```python
from build123d import *

# Parameters (mm, degrees)
F0_W     = 96.4296718666
F0_H     = 58.42
F1_DEPTH = 25.4
F4_DEPTH = 254
F6_DEPTH = 12.7
F2_R     = 8.8980244031
F7_DEPTH = 254


# Not quite as in the source:
# - a pattern or mirror of a feature is missing from the dataset's text; its kind, count and spacing are read off the source's solid


with BuildPart() as f1:
    # F0 (on Front) → F1 (new body, symmetric)
    with BuildSketch(Plane.XZ):
        Rectangle(F0_W, F0_H)
    extrude(amount=F1_DEPTH, both=True)

    # F3 (on face) → F4 (cut)
    with BuildSketch(Plane.XZ.offset(25.4)):
        with BuildLine():
            Line((12.7, 29.21), (-12.7, 29.21))
            ThreePointArc((-12.7, 29.21), (0, 16.51), (12.7, 29.21))
        make_face()
    extrude(amount=-F4_DEPTH, mode=Mode.SUBTRACT)

    # F5 (on face) → F6 (join)
    with BuildSketch(Plane(origin=(0, 25.4, 0), x_dir=(-1, 0, 0), z_dir=(0, 1, 0))):
        with BuildLine():
            Line((-12.7, 29.21), (-25.4, 29.21))
            ThreePointArc((-25.4, 29.21), (0, 3.81), (25.4, 29.21))
            Line((25.4, 29.21), (12.7, 29.21))
            ThreePointArc((12.7, 29.21), (0, 16.51), (-12.7, 29.21))
        make_face()
    f6 = extrude(amount=F6_DEPTH)

    # F6_copies: F6 across plane
    add(f6.mirror(Plane(origin=(0, 0, 0), x_dir=(0, 0, -1), z_dir=(0, -1, 0))))

    # F2 (on face) → F7 (cut)
    with BuildSketch(Plane.XY.offset(29.21)):
        with Locations((35.2072529495, 0)):
            Circle(F2_R)
        with Locations((-35.2072529495, 0)):
            Circle(F2_R)
    extrude(amount=-F7_DEPTH, mode=Mode.SUBTRACT)


solid = f1.part
```
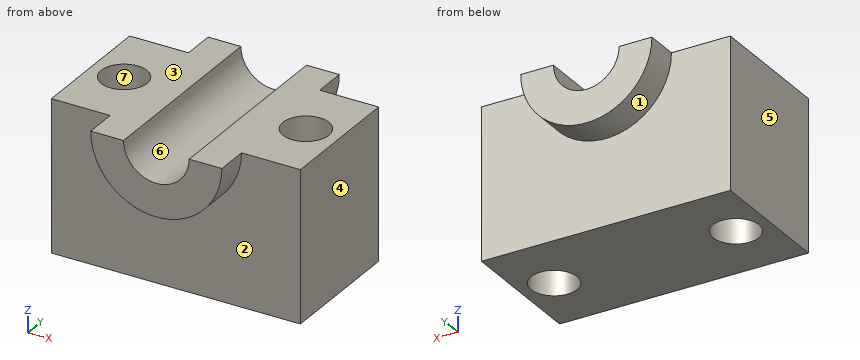
Check sheet for the modelled part. Datum: model origin and axes. Units: mm. Face numbers are marked on the shaded views. A direction names the side the tool comes from. Round coordinates to 2 decimals unless told otherwise and drop trailing zeros. Write each loop counter-clockwise with the first axis right and the second up, starting at its lowest first coordinate (ties: lowest second). Pieces come first, ordered by that corner, then holes. Notation, with made-up numbers: M 4,-10 L 35,-10 A29 cw 35,26 Z; hole C 46,38.5 d7. An arc over 180 degrees is marked long. Write item = value, one per line. Start each with the question number.
1. Section check D-D, the plane y = -20.5. Record the cut outline in (x, z).
2. Section check C-C, the plane x = 0. Record the cut outline in (y, z), then the cut area to 3 significant figures.
3. Gauge pin test, flat ends, axial feed: pin 1 (20.5 mm diameter, centred on x = -35.21, y = 0, fed in from -Z); pin 2 (8 mm diameter, centred on x = -35.5, y = -2, fed in from -Z); pin 3 (2 mm diameter, centred on y = -27, z = 6.5, fed in from +X); pin 4 (4 mm diameter, centred on x = 8, y = 23.5, fed in from +Z). Record the tip position at first contact, or that the pin passes through.
4. Section check B-B, the plane z = 2. Record the cut outline in (x, y), then the cut area to 3 significant figures.
5. Tool access check on the marked faces 1, 2 and 3. Record the directions out of +Z, -Z, +X, -X, +Y, -Y that give a thin tool (end or side, any length) a straight path to the whole face; none if there is none.
6. Release check for a two-part mould opening along X. For the marked faces 4, 5, 6 and 7 record: pulls with the +X half, pulls with the -X half, needs draft (parallel to the pull), parting line crosses it, or undercut.
7. Section check A-A, the plane y = 0. Record the cut outline in (x, z).
8. Scan lines: line 1 (X direction, y = 1.5, z = 1); line 2 (X direction, y = 0.5, z = 26.5); line 3 (X direction, y = -4.5, z = -0.5). Record each from-to range of solid material in increasing order. Write a range as [from, to].
Results found:
q1.outline = M -48.21,-29.21 L 48.21,-29.21 L 48.21,29.21 L 12.7,29.21 A12.7 cw -12.7,29.21 L -48.21,29.21 Z
q2.outline = M -38.1,3.81 L -25.4,3.81 L -25.4,-29.21 L 25.4,-29.21 L 25.4,3.81 L 38.1,3.81 L 38.1,16.51 L -38.1,16.51 Z
q2.area = 2,650 mm^2
q3.pin_1 = -29.21
q3.pin_2 = through
q3.pin_3 = 13.18
q3.pin_4 = 21.38
q4.outline = M -48.21,-25.4 L 48.21,-25.4 L 48.21,25.4 L -48.21,25.4 Z; hole C -35.21,0 d17.8; hole C 35.21,0 d17.8
q4.area = 4,400 mm^2
q5.face_1 = -Z, +Y
q5.face_2 = -Z, -Y
q5.face_3 = +Z, +X, -X, +Y, -Y
q6.face_4 = pulls with the +X half
q6.face_5 = pulls with the -X half
q6.face_6 = undercut
q6.face_7 = undercut
q7.outline = M -48.21,-29.21 L -44.11,-29.21 L -44.11,29.21 L -48.21,29.21 Z; M -26.31,-29.21 L 26.31,-29.21 L 26.31,29.21 L 12.7,29.21 A12.7 cw -12.7,29.21 L -26.31,29.21 Z; M 44.11,-29.21 L 48.21,-29.21 L 48.21,29.21 L 44.11,29.21 Z
q8.line_1 = [-48.21, -43.98], [-26.44, 26.44], [43.98, 48.21]
q8.line_2 = [-48.21, -44.09], [-26.32, -12.41], [12.41, 26.32], [44.09, 48.21]
q8.line_3 = [-48.21, -42.88], [-27.53, 27.53], [42.88, 48.21]
